Could you check a few things on this model? Use its own coordinates, in mm. A direction names the side the tool comes from. Give positions to 0.01 mm unless a question says otherwise; leave off trailing zeros. Loops run counter-clockwise (first coordinate to the right, second up) from the corner with the lowest first, then second, coordinate; pieces in that order, holes last. Notation, with made-up numbers: M -3,70.25 L 40,70.25 A19 ccw 40,88.25 Z; hole C 36,30 d6. An arc over 180 degrees is marked long. Return JSON: item names as keys, results as strings. Group by question number.
1. If we section it at C-C (y = 23.5): Write out the boundary of the cut face in (x, z).
2. If we section it at D-D (z = 25): Write out the boundary of the cut face in (x, y) (3 decimals).
3. For faces 4 (the flat face through (0, 13, 43)), 5 (the flat face through (-22.225, 13, 43)), which set-ups out of +Z, -Z, +X, -X, +Y, -Y let a thin tool reach every point of the face, with its end or its side?
4. If we section it at B-B (z = 12.7): Write out the boundary of the cut face in (x, y) (3 decimals), plus the area to 3 significant figures.
5. If we mould it in two halves opening along Y, with no side actions, what happens to faces 1 (the flat face through (-13, 25.4, 43)), 2 (the flat face through (-3.175, 13, 43)), 3 (the flat face through (-13, 0, 43))? For each: +Y half, -Y half, draft (parallel to the pull), parting line (faces both ways), or undercut.
6. Please list where these lines run through material, in increasing order: line 1 (Z direction, x = -12.7, y = 1.2); line 2 (X direction, y = 9.5, z = 38) (3 decimals); line 3 (Y direction, x = -4, z = 22) (3 decimals).
7. If we section it at A-A (y = 15.5): Write out the boundary of the cut face in (x, z) (3 decimals), plus the area to 3 significant figures.
Autodesk Inventor part; units mm, degrees
ref_plane "YZ Plane" through (0, 0, 0) normal (1, 0, 0) x (0, 1, 0)
ref_plane "XZ Plane" through (0, 0, 0) normal (0, 1, 0) x (-1, 0, 0)
ref_plane "XY Plane" through (0, 0, 0) normal (0, 0, 1) x (1, 0, 0)
sketch "Sketch1" plane through (0, 0, 0) normal (0, 0, 1) x (1, 0, 0)
  line L0 (0, 0) -> (-25.4, 0)
  line L1 (-25.4, 0) -> (-25.4, 25.4)
  line L2 (-25.4, 25.4) -> (0, 25.4)
  line L3 (0, 25.4) -> (0, 0)
  line L4 (-3.175, 22.225) -> (-22.225, 22.225)
  line L5 (-22.225, 22.225) -> (-22.225, 3.175)
  line L6 (-22.225, 3.175) -> (-3.175, 3.175)
  line L7 (-3.175, 3.175) -> (-3.175, 22.225)
  dimension "d0" = 25.4
  dimension "d1" = 25.4
  dimension "d2" = 3.175
extrude "Extrusion1" add sketch "Sketch1" along normal blind 86.36
sketch "Sketch2" plane through (-25.4, 25.4, 0) normal (0, 1, 0) x (1, 0, 0)
  line L0 (0, 0) -> (25.4, 0)
  line L1 (25.4, 0) -> (25.4, -86.36)
  line L2 (12.7, 0) -> (12.7, -12.7)
  circle A0 centre (12.7, -12.7) radius 3.3782
  dimension "d5" = 12.7
  dimension "d6" = 6.7564
extrude "Extrusion2" cut sketch "Sketch2" against normal blind 86.36
sketch "Sketch3" plane through (-25.4, 0, 0) normal (0, -1, 0) x (1, 0, 0)
  circle A0 centre (12.7, 73.66) radius 2.0701
  circle A1 centre (12.7, 60.96) radius 2.0701
  circle A2 centre (12.7, 48.26) radius 2.0701
  circle A3 centre (12.7, 35.56) radius 2.0701
extrude "Extrusion3" cut sketch "Sketch3" against normal blind 25.4
properties part number "side bumper mount" material "Aluminum 6061"
Answer:
{
 "1": {"outline": "M -25.4,0 L 0,0 L 0,86.36 L -25.4,86.36 Z; hole C -12.7,12.7 d6.76; hole C -12.7,35.56 d4.14; hole C -12.7,48.26 d4.14; hole C -12.7,60.96 d4.14; hole C -12.7,73.66 d4.14"},
 "2": {"outline": "M -25.4,0 L 0,0 L 0,25.4 L -25.4,25.4 Z; hole M -22.225,3.175 L -3.175,3.175 L -3.175,22.225 L -22.225,22.225 Z"},
 "3": {"face 4": "+Z, -Z, +X, +Y, -Y", "face 5": "+Z, -Z"},
 "4": {"outline": "M -25.4,0 L -16.078,0 L -16.078,3.175 L -22.225,3.175 L -22.225,22.225 L -16.078,22.225 L -16.078,25.4 L -25.4,25.4 Z; M -9.322,0 L 0,0 L 0,25.4 L -9.322,25.4 L -9.322,22.225 L -3.175,22.225 L -3.175,3.175 L -9.322,3.175 Z", "area": "239 mm²"},
 "5": {"face 1": "+Y half", "face 2": "undercut", "face 3": "-Y half"},
 "6": {"line 1": "z = 0 to 9.32, 16.08 to 33.49, 37.63 to 46.19, 50.33 to 58.89, 63.03 to 71.59, 75.73 to 86.36", "line 2": "x = -25.4 to -22.225, -3.175 to 0", "line 3": "y = 0 to 3.175, 22.225 to 25.4"},
 "7": {"outline": "M -25.4,0 L -22.225,0 L -22.225,86.36 L -25.4,86.36 Z; M -3.175,0 L 0,0 L 0,86.36 L -3.175,86.36 Z", "area": "548 mm²"}
}
